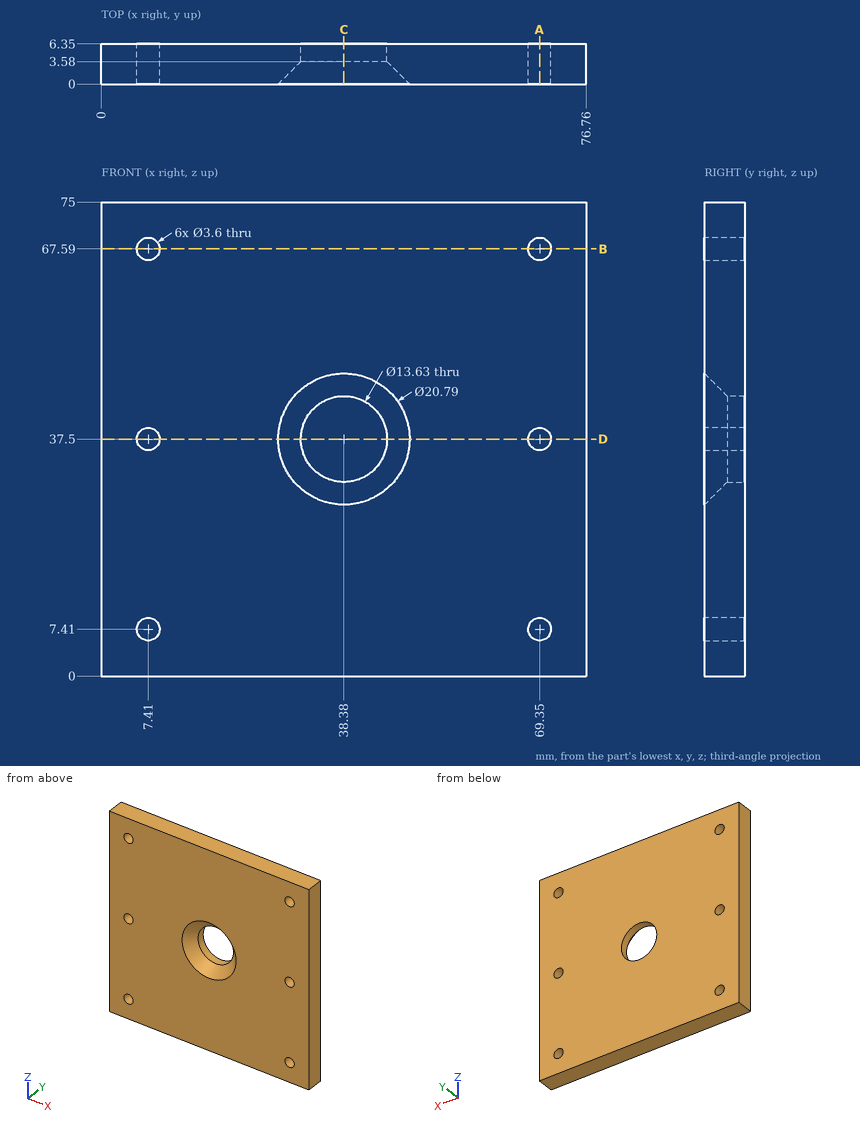
Check sheet for the drawn part. Datum: minimum x, y, z corner. Units: mm. Round coordinates to 2 decimals unless told otherwise and drop trailing zeros. Loops run counter-clockwise (first coordinate to the right, second up) from the corner with the lowest first, then second, coordinate; pieces in that order, holes last. Notation, with made-up numbers: (-15, -37) - (7, -37) arc R8 ccw to (7, -32) - close; hole circle Ø8 at (24.25, -35). An arc over 180 degrees is marked (long way). Answer as a JSON object with one key per item and string values. Group by question number.
Q1. Sectioned sample at C-C, the plane x = 38.38. Enter the section's corners in (y, z) (3 decimals).
Q2. Scan lines: line 1 along X through (y, z) = (5.25, 67.59); line 2 along Z through (x, y) = (69.35, 2.75); line 3 along X through (y, z) = (4, 37.5) (3 decimals). Record each from-to range of solid material in increasing order. Write a range as [from, to].
Q3. Sectioned sample at D-D, the plane z = 37.5. Enter the section's corners in (x, y) (3 decimals).
Q4. Sectioned sample at A-A, the plane x = 69.35. Enter the section's corners in (y, z), plus the area to 3 significant figures.
Q5. Sectioned sample at B-B, the plane z = 67.59. Enter the section's corners in (x, y).
Q6. Gauge pin test, flat end, axial feed: P1, Ø3, axis at x = 7.41, z = 7.41, coming from the -Y side. Record the tip position at first contact, or that the pin passes through.
Solution:
{
 "1": {"outline": "(0, 0) - (6.35, 0) - (6.35, 30.685) - (3.58, 30.685) - (0, 27.105) - close; (0, 47.895) - (3.58, 44.315) - (6.35, 44.315) - (6.35, 75) - (0, 75) - close"},
 "2": {"line 1": "x = [0, 5.61], [9.21, 67.55], [71.15, 76.76]", "line 2": "z = [0, 5.61], [9.21, 35.7], [39.3, 65.79], [69.39, 75]", "line 3": "x = [0, 5.61], [9.21, 31.565], [45.195, 67.55], [71.15, 76.76]"},
 "3": {"outline": "(0, 0) - (5.61, 0) - (5.61, 6.35) - (0, 6.35) - close; (9.21, 0) - (27.985, 0) - (31.565, 3.58) - (31.565, 6.35) - (9.21, 6.35) - close; (45.195, 3.58) - (48.775, 0) - (67.55, 0) - (67.55, 6.35) - (45.195, 6.35) - close; (71.15, 0) - (76.76, 0) - (76.76, 6.35) - (71.15, 6.35) - close"},
 "4": {"outline": "(0, 0) - (6.35, 0) - (6.35, 5.61) - (0, 5.61) - close; (0, 9.21) - (6.35, 9.21) - (6.35, 35.7) - (0, 35.7) - close; (0, 39.3) - (6.35, 39.3) - (6.35, 65.79) - (0, 65.79) - close; (0, 69.39) - (6.35, 69.39) - (6.35, 75) - (0, 75) - close", "area": "408 mm²"},
 "5": {"outline": "(0, 0) - (5.61, 0) - (5.61, 6.35) - (0, 6.35) - close; (9.21, 0) - (67.55, 0) - (67.55, 6.35) - (9.21, 6.35) - close; (71.15, 0) - (76.76, 0) - (76.76, 6.35) - (71.15, 6.35) - close"},
 "6": {"P1": "passes through"}
}
